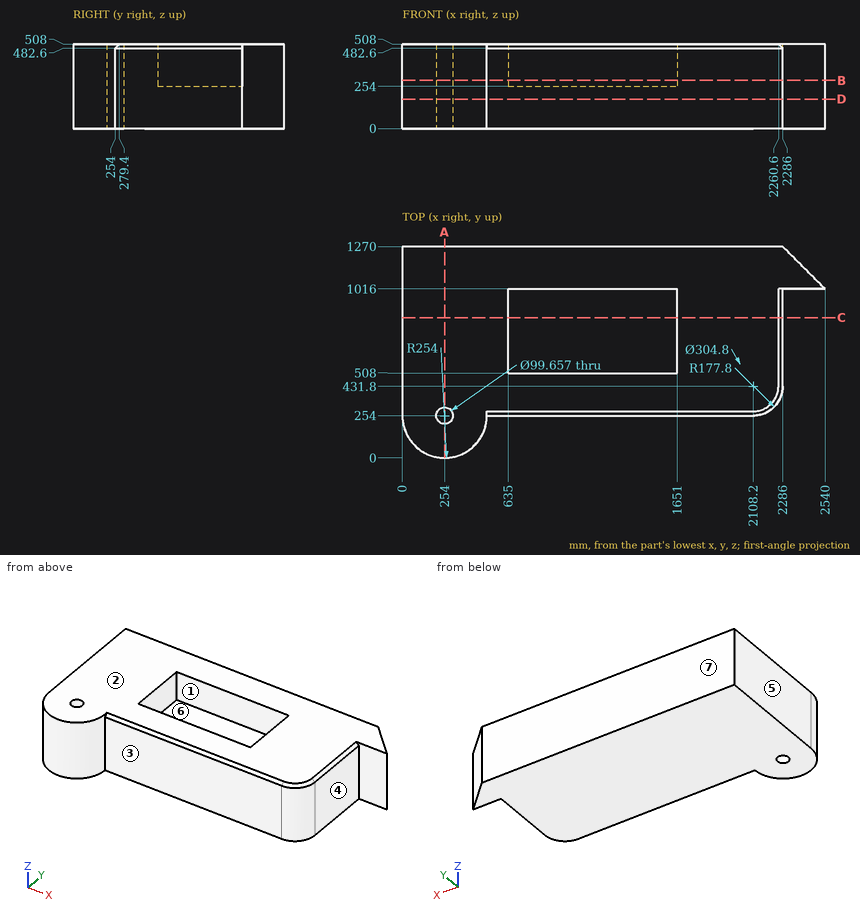
Could you check a few things on this drawing? It's one solid part, dimensions in mm from its lowest x, y, z. A direction names the side the tool comes from. Round coordinates to 2 decimals unless told otherwise and drop trailing zeros. Order: outer loops, then holes, each group sorted by start corner. A loop starts at its lowest first (then second) coordinate and runs counter-clockwise, first axis right, second up.
Q1. Imagine slicing it at B-B, the plane z = 289. List the corners of the cut face in (x, y) for me.
Geometry says:
outline: (0, 254) arc R254 ccw to (508, 254) - (2108.2, 254) arc R177.8 ccw to (2286, 431.8) - (2286, 1016) - (2540, 1016) - (2286, 1270) - (0, 1270) - close; hole circle Ø99.66 at (254, 254); hole (635, 508) - (1651, 508) - (1651, 1016) - (635, 1016) - close
Q2. Thinking about a two-plate mould opening in X: for the marked faces 4, 5, 6 and 7, which applies, released by +X, released by -X, zero draft, split by the parting line, or undercut?
Geometry says:
face 4: released by +X
face 5: released by -X
face 6: undercut
face 7: zero draft
Q3. I'm going to push flat-ended pins straight in: P1, Ø4, axis at y = 244.5, z = 51.5, coming from the -X side; P2, Ø4, axis at x = 326, z = 303.5, coming from the -Y side; P3, Ø4, axis at x = 1815.5, z = 59.5, coming from the -Y side. Where does each tip first touch, or does it pass through?
Geometry says:
P1: stops at x = 0.11
P2: stops at y = 9.84
P3: stops at y = 254
Q4. Please list where these lines run through material, in increasing order: probe 1 along Y at (x, z) = (254, 115); probe 2 along Y at (x, z) = (1485, 260); probe 3 along Z at (x, y) = (1058, 673).
Geometry says:
probe 1: y = 0 to 204.17, 303.83 to 1270
probe 2: y = 254 to 508, 1016 to 1270
probe 3: z = 0 to 254
Q5. Imagine slicing it at C-C, the plane y = 843.5. List the corners of the cut face in (x, z) for me.
Geometry says:
outline: (0, 0) - (2286, 0) - (2286, 482.6) - (2260.6, 508) - (1651, 508) - (1651, 254) - (635, 254) - (635, 508) - (0, 508) - close
Q6. Imagine slicing it at A-A, the plane x = 254. List the corners of the cut face in (y, z) for me.
Geometry says:
outline: (0, 0) - (204.17, 0) - (204.17, 508) - (0, 508) - close; (303.83, 0) - (1270, 0) - (1270, 508) - (303.83, 508) - close
Q7. Imagine slicing it at D-D, the plane z = 177. List the corners of the cut face in (x, y) for me.
Geometry says:
outline: (0, 254) arc R254 ccw to (508, 254) - (2108.2, 254) arc R177.8 ccw to (2286, 431.8) - (2286, 1016) - (2540, 1016) - (2286, 1270) - (0, 1270) - close; hole circle Ø99.66 at (254, 254)
Q8. Which directions (+Z, -Z, +X, -X, +Y, -Y) give clear straight access to the entire face, cutting with the end or side of a thin tool? Please do the marked faces 1, 2 and 3.
Geometry says:
face 1: +Z
face 2: +Z, +X, -X, +Y, -Y
face 3: +Z, -Z, +X, -Y
